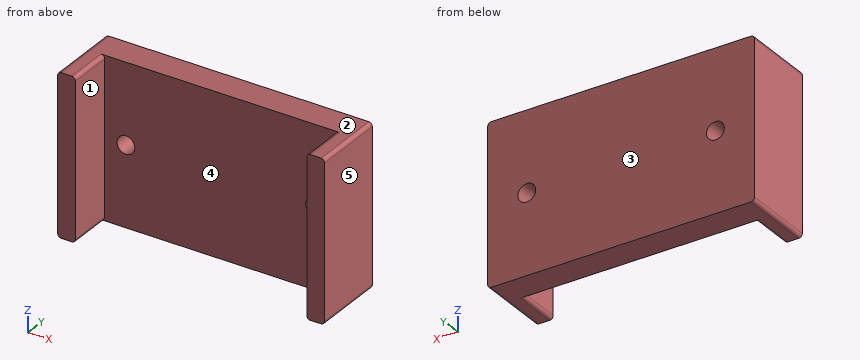
```python
from build123d import *

# Parameters (mm, degrees)
BOSS_EXTRUDE1_DEPTH = 45
SKETCH2_R           = 2.5
CUT_EXTRUDE1_DEPTH  = 89.345925203
FILLET1_R           = 1


with BuildPart() as part:
    # Sketch1 → Boss-Extrude1 (new body)
    with BuildSketch(Plane.XY):
        Polygon((0, 0), (5, 0), (5, 12.45), (70, 12.45), (70, 0), (75, 0), (75, 20.45), (0, 20.45), align=None)
    extrude(amount=BOSS_EXTRUDE1_DEPTH)

    # Sketch2 → Cut-Extrude1 (cut, through all)
    with BuildSketch(Plane.XZ.offset(-12.45)):
        with Locations(Location((11, 22.5, 0), (0, 0, 270))):
            Circle(SKETCH2_R)
        with Locations(Location((64, 22.5, 0), (0, 0, 270))):
            Circle(SKETCH2_R)
    extrude(amount=-CUT_EXTRUDE1_DEPTH, mode=Mode.SUBTRACT)

    # Fillet1
    fillet1_edges = [part.edges().sort_by_distance(p)[0] for p in [
        (5, 6.225, 0),
        (0, 10.225, 0),
        (5, 6.225, 45),
        (70, 6.225, 45),
        (75, 10.225, 45),
        (0, 10.225, 45),
        (75, 10.225, 0),
        (70, 6.225, 0),
    ]]
    fillet(fillet1_edges, radius=FILLET1_R)


solid = part.part
```
Geometry: final body of the model. Coordinates: model frame, mm. Face numbers are marked on the shaded views. A direction names the side the tool comes from. Coordinates: 2 decimals unless noted, no trailing zeros. Order: outer loops, then holes, each group sorted by start corner. A loop starts at its lowest first (then second) coordinate and runs counter-clockwise, first axis right, second up.
Item 1: Section query B-B (x = 11). Output: boundary loops of the cut face in (y, z), then the cut area to 3 significant figures.
Answer:
outline: (12.45, 0) - (20.45, 0) - (20.45, 20) - (12.45, 20) - close; (12.45, 25) - (20.45, 25) - (20.45, 45) - (12.45, 45) - close
area: 320 mm2
Item 2: Section query C-C (z = 22.5). Output: boundary loops of the cut face in (x, y).
Answer:
outline: (0, 0) - (5, 0) - (5, 12.45) - (8.5, 12.45) - (8.5, 20.45) - (0, 20.45) - close; (13.5, 12.45) - (61.5, 12.45) - (61.5, 20.45) - (13.5, 20.45) - close; (66.5, 12.45) - (70, 12.45) - (70, 0) - (75, 0) - (75, 20.45) - (66.5, 20.45) - close
Item 3: Section query D-D (z = 10). Output: boundary loops of the cut face in (x, y).
Answer:
outline: (0, 0) - (5, 0) - (5, 12.45) - (70, 12.45) - (70, 0) - (75, 0) - (75, 20.45) - (0, 20.45) - close
Item 4: Section query A-A (y = 3). Output: boundary loops of the cut face in (x, z), then the cut area to 3 significant figures.
Answer:
outline: (0, 1) arc R1 ccw to (1, 0) - (4, 0) arc R1 ccw to (5, 1) - (5, 44) arc R1 ccw to (4, 45) - (1, 45) arc R1 ccw to (0, 44) - close; (70, 1) arc R1 ccw to (71, 0) - (74, 0) arc R1 ccw to (75, 1) - (75, 44) arc R1 ccw to (74, 45) - (71, 45) arc R1 ccw to (70, 44) - close
area: 448 mm2
Item 5: Access query for the marked faces 1 and 2. Directions: +Z, -Z, +X, -X, +Y, -Y. A direction counts if a zero-diameter tool reaches every point of the face in a straight line with its end or side. Return the directions, or none.
Answer:
face 1: +Z, -Z, -Y
face 2: +Z, +X, -X, +Y, -Y
Item 6: Material intervals for line 1 along X through (y, z) = (16.25, 22.5); line 2 along X through (y, z) = (12, 15.5); line 3 along Y through (x, z) = (45.5, 16.5), sorted ascending.
Answer:
line 1: x = 0 to 8.5, 13.5 to 61.5, 66.5 to 75
line 2: x = 0 to 5, 70 to 75
line 3: y = 12.45 to 20.45
Item 7: Contact query for a flat-ended pin moving along its axis: P1, Ø13.5, axis at x = 48.5, z = 19, coming from the -Y side. Output: stop coordinate, or through.
Answer:
P1: stops at y = 12.45
Item 8: Draft query along X for the marked faces 3, 4 and 5. Return one class per face: released by +X, released by -X, zero draft, split by the parting line, or undercut.
Answer:
face 3: zero draft
face 4: undercut
face 5: released by +X
